Work out the finished part from the listing and answer in its coordinate system (mm). Face numbers are marked on the shaded views. A direction names the side the tool comes from. Round coordinates to 2 decimals unless told otherwise and drop trailing zeros. Order: outer loops, then holes, each group sorted by start corner. A loop starts at its lowest first (then second) coordinate and runs counter-clockwise, first axis right, second up. Notation, with made-up numbers: (-11.75, -8) - (29.25, -8) arc R13 ccw to (29.25, 8) - close; hole circle Ø4 at (-12.75, 1). An arc over 180 degrees is marked (long way). Answer in a Markdown table with one row per item.
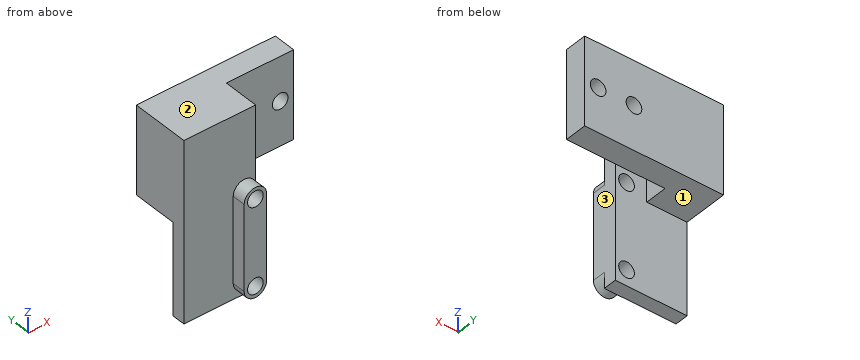
from build123d import *

# Parameters (mm, degrees)
F0_W      = 16
F0_H      = 40
F0_R      = 1.75
F1_DEPTH  = 3
F2_R      = 1.75
F3_DEPTH  = 3
F4_W      = 16
F4_H      = 19.6
F4_R      = 1.75
F5_DEPTH  = 10
F6_W      = 5
F6_H      = 19.6
F7_DEPTH  = 15
F8_R      = 1.75
F9_DEPTH  = 5
F10_W     = 7
F10_H     = 5
F11_DEPTH = 7
F12_R     = 1.75
F13_DEPTH = 5


with BuildPart() as f1:
    # F0 (on Front) → F1 (new body)
    with BuildSketch(Plane.XZ):
        with Locations((8, 20)):
            Rectangle(F0_W, F0_H)
        with Locations((13.5, 3.5)):
            Circle(F0_R, mode=Mode.SUBTRACT)
        with Locations((13.5, 22.5)):
            Circle(F0_R, mode=Mode.SUBTRACT)
    extrude(amount=F1_DEPTH)

    # F2 (on face) → F3 (join)
    with BuildSketch(Plane.XZ.offset(3)):
        with BuildLine():
            ThreePointArc((11, 3.5), (13.5, 1), (16, 3.5))
            Line((16, 3.5), (16, 22.5))
            ThreePointArc((16, 22.5), (13.5, 25), (11, 22.5))
            Line((11, 22.5), (11, 3.5))
        make_face()
        with Locations((13.5, 3.5)):
            Circle(F2_R, mode=Mode.SUBTRACT)
        with Locations((13.5, 22.5)):
            Circle(F2_R, mode=Mode.SUBTRACT)
    extrude(amount=F3_DEPTH)

    # F4 (on face) → F5 (join)
    with BuildSketch(Plane(origin=(0, 0, 0), x_dir=(-1, 0, 0), z_dir=(0, 1, 0))):
        with Locations((-8, 30.2)):
            Rectangle(F4_W, F4_H)
        with Locations((-13.5, 22.5)):
            Circle(F4_R, mode=Mode.SUBTRACT)
    extrude(amount=F5_DEPTH)

    # F6 (on face) → F7 (join)
    with BuildSketch(Plane.YZ.offset(16)):
        with Locations((7.5, 30.2)):
            Rectangle(F6_W, F6_H)
    extrude(amount=F7_DEPTH)

    # F8 (on face) → F9 (cut, through all)
    with BuildSketch(Plane.XZ.offset(-5)):
        with Locations((20, 30.2)):
            Circle(F8_R)
        with Locations((28, 30.2)):
            Circle(F8_R)
    extrude(amount=-F9_DEPTH, mode=Mode.SUBTRACT)

    # F10 (on face) → F11 (cut)
    with BuildSketch(Plane(origin=(0, 0, 20.4), x_dir=(1, 0, 0), z_dir=(0, 0, -1))):
        with Locations((12.5, -2.5)):
            Rectangle(F10_W, F10_H)
    extrude(amount=-F11_DEPTH, mode=Mode.SUBTRACT)

    # F12 (on face) → F13 (join, through all)
    with BuildSketch(Plane.XZ.offset(-5)):
        with Locations((13.5, 22.5)):
            Circle(F12_R)
    extrude(amount=-F13_DEPTH)


solid = f1.part
1) Find section C-C, the plane y = -0.75. Give the vertices of the cut face in (x, z), then the cut area to 3 significant figures.
Filled in:
| item | result |
|---|---|
| outline | (0, 0) - (16, 0) - (16, 40) - (0, 40) - close; hole circle Ø3.5 at (13.5, 3.5); hole circle Ø3.5 at (13.5, 22.5) |
| area | 621 mm^2 |
2) Find section A-A, the plane x = 28. Give the vertices of the cut face in (y, z).
Filled in:
| item | result |
|---|---|
| outline | (5, 20.4) - (10, 20.4) - (10, 28.45) - (5, 28.45) - close; (5, 31.95) - (10, 31.95) - (10, 40) - (5, 40) - close |
3) Each of these flat-tipped pins is pushed along its axis until it touches: pin 1 (2 mm diameter, centred on x = 18.5, z = 9, fed in from -Y); pin 2 (4 mm diameter, centred on x = 20, z = 30.2, fed in from -Y); pin 3 (4.5 mm diameter, centred on x = 13.5, z = 3.5, fed in from -Y); pin 4 (17.5 mm diameter, centred on x = 7.5, z = 10, fed in from +Y). Where does it stop, or does it pass through?
Filled in:
| item | result |
|---|---|
| pin 1 | passes through |
| pin 2 | stops at y = 5 |
| pin 3 | stops at y = -6 |
| pin 4 | stops at y = 0 |
4) Find section B-B, the plane z = 30.2. Give the vertices of the cut face in (x, y), then the cut area to 3 significant figures.
Filled in:
| item | result |
|---|---|
| outline | (0, -3) - (16, -3) - (16, 5) - (18.25, 5) - (18.25, 10) - (0, 10) - close; (21.75, 5) - (26.25, 5) - (26.25, 10) - (21.75, 10) - close; (29.75, 5) - (31, 5) - (31, 10) - (29.75, 10) - close |
| area | 248 mm^2 |
5) Find the intervals of material crossed by probe 1 along Z at (x, y) = (13.5, -1.5); probe 2 along Z at (x, y) = (28, 7.3); probe 3 along X at (y, z) = (4.5, 29), in increasing order. Write a range as from..to.
Filled in:
| item | result |
|---|---|
| probe 1 | z = 0..1.75, 5.25..20.75, 24.25..40 |
| probe 2 | z = 20.4..28.45, 31.95..40 |
| probe 3 | x = 0..16 |
6) Which of the six approach directions +Z, -Z, +X, -X, +Y, -Y give full straight-line access (tool end or side, diameter ignored) to the marked faces 1, 2 and 3?
Filled in:
| item | result |
|---|---|
| face 1 | -Z, +X, -X, +Y |
| face 2 | +Z, +X, -X, +Y, -Y |
| face 3 | +Z, -Z, +X, -Y |
7) Find section D-D, the plane x = 13.5. Give the vertices of the cut face in (y, z).
Filled in:
| item | result |
|---|---|
| outline | (-6, 1) - (-3, 1) - (-3, 0) - (0, 0) - (0, 1.75) - (-6, 1.75) - close; (-6, 5.25) - (0, 5.25) - (0, 20.75) - (-6, 20.75) - close; (-6, 24.25) - (0, 24.25) - (0, 27.4) - (5, 27.4) - (5, 20.4) - (10, 20.4) - (10, 40) - (-3, 40) - (-3, 25) - (-6, 25) - close |
